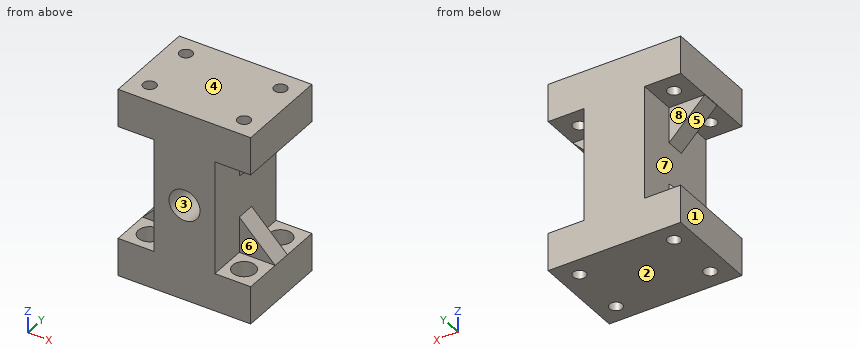
```python
from build123d import *

# Parameters (mm, degrees)
SKETCH2_R           = 1.7
BOSS_EXTRUDE1_DEPTH = 50
CUT_EXTRUDE1_DEPTH  = 51
CUT_EXTRUDE2_START  = -22.181644
SKETCH4_R           = 4.1
CUT_EXTRUDE2_DEPTH  = 22.181644
CUT_EXTRUDE3_START  = -6
SKETCH6_R           = 3
SKETCH6_R_2         = 1.7
CUT_EXTRUDE3_DEPTH  = 6
BOSS_EXTRUDE2_DEPTH = 2.5


with BuildPart() as part:
    # Sketch2 → Boss-Extrude1 (new body)
    with BuildSketch(Plane.XY):
        Polygon((29.223766163, 230.865012057), (29.223766163, 235.92362241), (24.223766163, 235.92362241), (-0.776233837, 235.92362241), (-5.776233837, 235.92362241), (-5.776233837, 230.92362241), (-5.776233837, 210.982238102), (24.223766163, 210.982238102), (29.223766163, 210.982238102), (29.223766163, 215.982238102), align=None)
        with Locations((-0.776233837, 216.130599455)):
            Circle(SKETCH2_R, mode=Mode.SUBTRACT)
        with Locations((24.223766163, 215.982238102)):
            Circle(SKETCH2_R, mode=Mode.SUBTRACT)
        with Locations((-0.776233837, 230.92362241)):
            Circle(SKETCH2_R, mode=Mode.SUBTRACT)
        with Locations((24.223766163, 230.865012057)):
            Circle(SKETCH2_R, mode=Mode.SUBTRACT)
    extrude(amount=BOSS_EXTRUDE1_DEPTH)

    # Sketch3 → Cut-Extrude1 (cut)
    with BuildSketch(Plane(origin=(0, 235.92362241, 0), x_dir=(1, 0, 0), z_dir=(0, 1, 0))):
        Polygon((3.750473292, -40), (3.750473292, -27), (3.750473292, -10), (-5.776233837, -10), (-5.776233837, -40), align=None)
        Polygon((29.223766163, -10), (19.750473292, -10), (19.750473292, -27), (19.750473292, -40), (29.223766163, -40), align=None)
    extrude(amount=-CUT_EXTRUDE1_DEPTH, mode=Mode.SUBTRACT)

    # Sketch4 → Cut-Extrude2 (cut)
    with BuildSketch(Plane.XZ.offset(-210.982238102).offset(CUT_EXTRUDE2_START)):
        with Locations(Location((11.743125017, 25.37, 0), (0, 0, 270))):
            Circle(SKETCH4_R)
    extrude(amount=CUT_EXTRUDE2_DEPTH, mode=Mode.SUBTRACT)

    # Sketch6 → Cut-Extrude3 (cut)
    # profile 1 of 4: a face of its own
    with BuildSketch(Plane.XY.offset(10).offset(CUT_EXTRUDE3_START)):
        with Locations((24.223766163, 230.865012057)):
            Circle(SKETCH6_R)
    # profile 2 of 4: a face of its own
    with BuildSketch(Plane.XY.offset(10).offset(CUT_EXTRUDE3_START)):
        with Locations((24.223766163, 215.982238102)):
            Circle(SKETCH6_R)
        with Locations((24.223766163, 215.982238102)):
            Circle(SKETCH6_R_2, mode=Mode.SUBTRACT)
    # profile 3 of 4: a face of its own
    with BuildSketch(Plane.XY.offset(10).offset(CUT_EXTRUDE3_START)):
        with Locations((-0.776233837, 216.130599455)):
            Circle(SKETCH6_R)
        with Locations((-0.776233837, 216.130599455)):
            Circle(SKETCH6_R_2, mode=Mode.SUBTRACT)
    # profile 4 of 4: a face of its own
    with BuildSketch(Plane.XY.offset(10).offset(CUT_EXTRUDE3_START)):
        with Locations((-0.776233837, 230.92362241)):
            Circle(SKETCH6_R)
        with Locations((-0.776233837, 230.92362241)):
            Circle(SKETCH6_R_2, mode=Mode.SUBTRACT)
    extrude(amount=CUT_EXTRUDE3_DEPTH, mode=Mode.SUBTRACT)

    # Sketch8 → Boss-Extrude2 (add, symmetric)
    with BuildSketch(Plane(origin=(0, 223.452930256, 0), x_dir=(1, 0, 0), z_dir=(0, 1, 0))):
        Polygon((3.750473292, -30.597830669), (-5.651696039, -40), (3.750473292, -40), align=None)
        Polygon((19.750473292, -40), (29.223766163, -40), (19.750473292, -30.52670713), align=None)
        Polygon((19.750473292, -10), (19.750473292, -19.47329287), (29.223766163, -10), align=None)
        Polygon((3.750473292, -10), (-5.776233837, -10), (3.750473292, -19.52670713), align=None)
    extrude(amount=BOSS_EXTRUDE2_DEPTH, both=True)


solid = part.part
```
For this review, take the finished solid that the model builds, in its own axes (mm). Face numbers are marked on the shaded views. A direction names the side the tool comes from. Coordinates: 2 decimals unless noted, no trailing zeros. Order: outer loops, then holes, each group sorted by start corner. A loop starts at its lowest first (then second) coordinate and runs counter-clockwise, first axis right, second up. Notation, with made-up numbers: (-25, -28.75) -> (-7, -28.75) arc R14 cw to (-7, -15.75) -> close; hole circle Ø11 at (-25.75, -29.75). An arc over 180 degrees is marked (long way). Use CSV: the item, a comma, the result in double quotes. Start each with the question number.
Item 1: We need section B-B, the plane y = 228.5. Give the boundary of the cut face in (x, z), then the cut area to 3 significant figures.
Item 2: Draft analysis for pull direction Z (two halves, no side actions). For the marked faces 1, 2, 3 and 4, state which applies: pulls with the +Z half, pulls with the -Z half, needs draft (parallel to the pull), parting line crosses it, or undercut.
Item 3: We need section A-A, the plane z = 25.37. Give the boundary of the cut face in (x, y).
Item 4: For the marked faces 5, 6, 7 and 8, list the 3-axis set-ups (+Z, -Z, +X, -X, +Y, -Y) from which the entire face can be reached by the end or side of a thin tool; tool diameter is ignored.
Item 5: We need section D-D, the plane y = 220.25. Give the boundary of the cut face in (x, z), then the cut area to 3 significant figures.
Item 6: Insertion check: pin 1 (2 mm diameter, centred on x = 0.5, z = 16.5, fed in from -Y); pin 2 (2 mm diameter, centred on y = 220.5, z = 14, fed in from +X); pin 3 (4.5 mm diameter, centred on x = -2.5, z = 34, fed in from +Y). Each pin has a flat end and moves straight along its axis. Give the tip position at first contact, or say it passes through.
Item 7: Wall thickness on probe 1 along Z at (x, y) = (11.5, 225.5); probe 2 along Y at (x, z) = (26, 5); probe 3 along X at (y, z) = (220, 27): over which ranges is each line inside the solid? List them lowest first.
Item 8: We need section C-C, the plane x = 8.5. Give the boundary of the cut face in (y, z).
Derived:
1,outline,"(-5.78, 0) -> (29.22, 0) -> (29.22, 10) -> (26.07, 10) -> (26.07, 4) -> (22.38, 4) -> (22.38, 10) -> (19.75, 10) -> (19.75, 40) -> (29.22, 40) -> (29.22, 50) -> (-5.78, 50) -> (-5.78, 40) -> (3.75, 40) -> (3.75, 10) -> (0.99, 10) -> (0.99, 4) -> (-2.54, 4) -> (-2.54, 10) -> (-5.78, 10) -> close; hole circle Ø8.2 at (11.74, 25.37)"
1,area,"1,080 mm^2"
2,face 1,"needs draft"
2,face 2,"pulls with the -Z half"
2,face 3,"undercut"
2,face 4,"pulls with the +Z half"
3,outline,"(3.75, 210.98) -> (7.64, 210.98) -> (7.64, 233.16) -> (15.84, 233.16) -> (15.84, 210.98) -> (19.75, 210.98) -> (19.75, 235.92) -> (3.75, 235.92) -> close"
4,face 5,"-X, +Y, -Y"
4,face 6,"+X, -Y"
4,face 7,"-X"
4,face 8,"-X, +Y"
5,outline,"(-5.78, 0) -> (29.22, 0) -> (29.22, 10) -> (19.75, 10) -> (19.75, 40) -> (29.22, 40) -> (29.22, 50) -> (-5.78, 50) -> (-5.78, 40) -> (3.75, 40) -> (3.75, 10) -> (-5.78, 10) -> close; hole circle Ø8.2 at (11.74, 25.37)"
5,area,"1,130 mm^2"
6,pin 1,"stops at y = 220.95"
6,pin 2,"stops at x = 26.12"
6,pin 3,"stops at y = 225.95"
7,probe 1,"z = 0 to 21.28, 29.46 to 50"
7,probe 2,"y = 210.98 to 213.56, 218.4 to 228.45, 233.28 to 235.92"
7,probe 3,"x = 3.75 to 7.98, 15.51 to 19.75"
8,outline,"(210.98, 0) -> (235.92, 0) -> (235.92, 50) -> (210.98, 50) -> (210.98, 27.88) -> (233.16, 27.88) -> (233.16, 22.86) -> (210.98, 22.86) -> close"
